Build history of the part. All positions in model axes, mm. A direction names the side the tool comes from. Give positions to 0.01 mm unless a question says otherwise; leave off trailing zeros. Loops run counter-clockwise (first coordinate to the right, second up) from the corner with the lowest first, then second, coordinate; pieces in that order, holes last. Notation, with made-up numbers: M 56.5,37.25 L 80.5,37.25 A19 ccw 80.5,62.25 Z; hole C 24,5.5 d8. An arc over 180 degrees is marked long. Answer as a JSON object with one key per item and string values. Group by question number.
1. Drop flat-ended pins along their axis: pin 1 Ø1 at (y, z) = (-6, 26.35) entering from -X; pin 2 Ø1.8 at (x, z) = (4.95, 20.95) entering from -Y; pin 3 Ø1 at (x, z) = (17, 14) entering from -Y; pin 4 Ø4 at (x, z) = (-2.5, 14.5) entering from +Y. Give the stop position or say it passes through.
2. Slice it at B-B (x = 0). List the corners of the cut face in (y, z), then the cut area to 3 significant figures.
3. Drill centre lines: line 1 along X through (y, z) = (-5, 27.25); line 2 along Y through (x, z) = (17.05, 5.65); line 3 along Y through (x, z) = (-0.5, 6.5). Where is each one in solid material? Low to high. Write a range as [from, to].
4. Slice it at C-C (z = 16). List the corners of the cut face in (x, y).
5. 3-axis set-ups, long thin cutter, end or side, ignore diameter. For faces 4 (the face through (-4, 0, 18)), 5 (the face through (-17.014, -4.756, 22.815)): which of +Z, -Z, +X, -X, +Y, -Y reach the whole face in a straight line?
6. Slice it at A-A (z = 5.65). List the corners of the cut face in (x, y), then the cut area to 3 significant figures.
7. Mould opens along X. For faces 1 (the face through (4.24, -0.99, 11.42)), 2 (the face through (-17, -7.455, 6)), 3 (the face through (18, -3, 16)) say: released by +X, released by -X, zero draft, split by the parting line, or undercut.
8. Slice it at D-D (x = 11). List the corners of the cut face in (y, z), then the cut area to 3 significant figures.
from build123d import *

# Parameters (mm, degrees)
EXTRUDE_1_DEPTH     = 32
FILLET_1_R          = 1
SKETCH_2_R          = 0.8
CUT_EXTRUDE_1_DEPTH = 50.085647116
SKETCH_3_W          = 43.847258393
SKETCH_3_H          = 18.19729806
CUT_EXTRUDE_2_DEPTH = 4
SKETCH_4_W          = 47.825059727
SKETCH_4_H          = 17.237139118
CUT_EXTRUDE_3_DEPTH = 4
SKETCH_5_W          = 40.336284727
SKETCH_5_H          = 27.150302887
CUT_EXTRUDE_4_DEPTH = 2
SKETCH_6_W          = 15
SKETCH_6_H          = 3
CUT_EXTRUDE_5_DEPTH = 47.212335629
FILLET_2_R          = 1
SKETCH_7_R          = 4
SKETCH_7_R_2        = 0.8
CUT_EXTRUDE_6_DEPTH = 2


with BuildPart() as part:
    # 草图1 → 凸台-拉伸1 (new body)
    with BuildSketch(Plane.XY):
        Polygon((-18, 0), (18, 0), (18, -9.455197133), (16, -9.455197133), (16, -2), (-16, -2), (-16, -8.573476703), (-18, -8.573476703), align=None)
    extrude(amount=EXTRUDE_1_DEPTH)

    # 圆角1
    fillet_1_edges = [part.edges().sort_by_distance(p)[0] for p in [
        (-18, 0, 16),
        (18, 0, 16),
        (16, -2, 16),
        (-16, -2, 16),
    ]]
    fillet(fillet_1_edges, radius=FILLET_1_R)

    # 草图2 → 切除-拉伸1 (cut, through all)
    with BuildSketch(Plane(origin=(18, 0, 0), x_dir=(0, 0, -1), z_dir=(1, 0, 0))):
        with Locations((-26.35, -6)):
            Circle(SKETCH_2_R)
        with Locations((-5.65, -6)):
            Circle(SKETCH_2_R)
    extrude(amount=-CUT_EXTRUDE_1_DEPTH, mode=Mode.SUBTRACT)

    # 草图3 → 切除-拉伸2 (cut)
    with BuildSketch(Plane.XY.offset(32)):
        with Locations((-0.045721854, -4.064631677)):
            Rectangle(SKETCH_3_W, SKETCH_3_H)
    extrude(amount=-CUT_EXTRUDE_2_DEPTH, mode=Mode.SUBTRACT)

    # 草图4 → 切除-拉伸3 (cut)
    with BuildSketch(Plane(origin=(0, 0, 0), x_dir=(-1, 0, 0), z_dir=(0, 0, -1))):
        with Locations((0.800132453, -3.310221079)):
            Rectangle(SKETCH_4_W, SKETCH_4_H)
    extrude(amount=-CUT_EXTRUDE_3_DEPTH, mode=Mode.SUBTRACT)

    # 草图5 → 切除-拉伸4 (cut)
    with BuildSketch(Plane.XZ.offset(9.455197133)):
        with Locations((0.686769888, 16.04578466)):
            Rectangle(SKETCH_5_W, SKETCH_5_H)
    extrude(amount=-CUT_EXTRUDE_4_DEPTH, mode=Mode.SUBTRACT)

    # 草图6 → 切除-拉伸5 (cut, through all)
    with BuildSketch(Plane(origin=(18, 0, 0), x_dir=(0, 0, -1), z_dir=(1, 0, 0))):
        with Locations((-15.6, -5.955197133)):
            Rectangle(SKETCH_6_W, SKETCH_6_H)
    extrude(amount=-CUT_EXTRUDE_5_DEPTH, mode=Mode.SUBTRACT)

    # 圆角2
    fillet_2_edges = [part.edges().sort_by_distance(p)[0] for p in [
        (-17, -7.455197133, 4),
        (17, -7.455197133, 4),
        (17, -7.455197133, 28),
        (-17, -7.455197133, 28),
        (17, -7.455197133, 8.1),
        (17, -7.455197133, 23.1),
        (-17, -4.455197133, 23.1),
        (17, -4.455197133, 23.1),
        (-17, -7.455197133, 8.1),
        (-17, -7.455197133, 23.1),
        (-17, -4.455197133, 8.1),
        (17, -4.455197133, 8.1),
    ]]
    fillet(fillet_2_edges, radius=FILLET_2_R)

    # 草图7 → 切除-拉伸6 (cut)
    with BuildSketch(Plane(origin=(0, 0, 0), x_dir=(1, 0, 0), z_dir=(0, 1, 0))):
        with Locations(Location((0, -16, 0), (0, 0, 270))):
            Circle(SKETCH_7_R)
        with Locations(Location((4.949747468, -11.050252532, 0), (0, 0, 270))):
            Circle(SKETCH_7_R_2)
        with Locations(Location((4.949747468, -20.949747468, 0), (0, 0, 270))):
            Circle(SKETCH_7_R_2)
        with Locations(Location((-4.949747468, -20.949747468, 0), (0, 0, 270))):
            Circle(SKETCH_7_R_2)
        with Locations(Location((-4.949747468, -11.050252532, 0), (0, 0, 270))):
            Circle(SKETCH_7_R_2)
    extrude(amount=-CUT_EXTRUDE_6_DEPTH, mode=Mode.SUBTRACT)


solid = part.part
Established:
{
 "1": {"pin 1": "passes through", "pin 2": "stops at y = -2", "pin 3": "stops at y = -4.46", "pin 4": "stops at y = 0"},
 "2": {"outline": "M -2,4 L 0,4 L 0,12 L -2,12 Z; M -2,20 L 0,20 L 0,28 L -2,28 Z", "area": "32.0 mm^2"},
 "3": {"line 1": "x = [-18, -16], [16, 18]", "line 2": "y = [-7.46, -6.8], [-5.2, 0]", "line 3": "y = [-2, 0]"},
 "4": {"outline": "M -18,-4.46 L -16,-4.46 L -16,-3 A1 cw -15,-2 L -4,-2 L -4,0 L -17,0 A1 ccw -18,-1 Z; M 4,-2 L 15,-2 A1 cw 16,-3 L 16,-4.46 L 18,-4.46 L 18,-1 A1 ccw 17,0 L 4,0 Z"},
 "5": {"face 4": "+Z, -Z, +X, -X, +Y", "face 5": "+X, -X, -Y"},
 "6": {"outline": "M -18,-7.46 L -16,-7.46 L -16,-6.8 L -18,-6.8 Z; M -18,-5.2 L -16,-5.2 L -16,-3 A1 cw -15,-2 L 15,-2 A1 cw 16,-3 L 16,-5.2 L 18,-5.2 L 18,-1 A1 ccw 17,0 L -17,0 A1 ccw -18,-1 Z; M 16,-7.46 L 18,-7.46 L 18,-6.8 L 16,-6.8 Z", "area": "87.4 mm^2"},
 "7": {"face 1": "undercut", "face 2": "zero draft", "face 3": "released by +X"},
 "8": {"outline": "M -2,4 L 0,4 L 0,28 L -2,28 Z", "area": "48.0 mm^2"}
}
